Verification items for the finished model (mm, model axes). A direction names the side the tool comes from. Give positions to 0.01 mm unless a question says otherwise; leave off trailing zeros. Write each loop counter-clockwise with the first axis right and the second up, starting at its lowest first coordinate (ties: lowest second). Pieces come first, ordered by that corner, then holes.
Autodesk Inventor part; units mm, degrees
ref_plane "YZ Plane" through (0, 0, 0) normal (1, 0, 0) x (0, 1, 0)
ref_plane "XZ Plane" through (0, 0, 0) normal (0, 1, 0) x (-1, 0, 0)
ref_plane "XY Plane" through (0, 0, 0) normal (0, 0, 1) x (1, 0, 0)
sketch "Sketch1" plane through (0, 0, 0) normal (0, 0, 1) x (1, 0, 0)
  circle A0 centre (12.5, 11.5) radius 1.6
  line L0 (0, 0) -> (18, 0)
  line L1 (0, 0) -> (0, 3)
  arc A1 (18, 11.5) -> (7.7369, 14.25) centre (12.5, 11.5) ccw
  line L2 (12.5, 11.5) -> (7.7369, 14.25) construction
  line L3 (12.5, 11.5) -> (18, 11.5) construction
  line L4 (7.7369, 14.25) -> (0, 3)
  line L5 (18, 11.5) -> (18, 0)
  dimension "d17" = 3
  dimension "d19" = 11.5
  dimension "d23" = 90
  dimension "d25" = 12.5
  dimension "d31" = 5.5
  dimension "d32" = 150
  dimension "d49" = 3.2
extrude "Extrusion1" add sketch "Sketch1" along normal blind 4.5
sketch "Sketch4" plane through (0, 0, 4.5) normal (0, 0, 1) x (1, 0, 0)
  line L0 (0, 3) -> (0, 0)
  line L1 (18, 0) -> (18, 3)
  line L2 (0, 0) -> (18, 0)
  line L3 (18, 0) -> (18, 3)
  line L4 (18, 3) -> (0, 3)
  line L5 (0, 3) -> (0, 0)
  line L6 (18, 0) -> (18, 11.5)
extrude "Extrusion2" add sketch "Sketch4" along normal blind 4.5
sketch "Sketch5" plane through (0, 0, 0) normal (0, -1, 0) x (1, 0, 0)
  circle A0 centre (5, 5) radius 1.6
  circle A1 centre (15, 5) radius 1.6
  line L0 (0, 0) -> (18, 0)
  point P0 (20.0001, 0)
  dimension "d13" = 3.2
  dimension "d14" = 3.2
  dimension "d38" = 5
  dimension "d39" = 5
extrude "Extrusion3" cut sketch "Sketch5" against normal through all
sketch "Sketch6" plane through (0, 3, 9) normal (0, 1, 0) x (1, 0, 0)
  circle A0 centre (5, 4) radius 1.6
  circle A1 centre (5, 4) radius 3
  circle A2 centre (15, 4) radius 1.6
  circle A3 centre (15, 4) radius 3
  line L0 (0, 9) -> (18, 9)
  point P0 (20.0001, 9)
  dimension "d34" = 6
  dimension "d35" = 6
  dimension "d40" = 5
  dimension "d41" = 5
extrude "Extrusion4" cut sketch "Sketch6" along normal up to next
sketch "Sketch7" plane through (0, 0, 0) normal (0, -1, 0) x (1, 0, 0)
  line L0 (0, 0) -> (0, 9)
  line L1 (2.042, 0) -> (0, 0)
  line L2 (0, 0) -> (0, 9)
  line L3 (0, 9) -> (2.042, 9)
  line L4 (2.042, 9) -> (2.042, 0)
extrude "Extrusion5" cut sketch "Sketch7" against normal up to next
properties part number "lower_deck_shaft_mount_v3_for_AD"
Item 1: Scan lines: line 1 along Z through (x, y) = (15, 1.35); line 2 along Y through (x, z) = (12.5, 1.8); line 3 along Z through (x, y) = (11.25, 4.75). Record each from-to range of solid material in increasing order.
Answer key:
line 1: z = 0 to 3.4, 6.6 to 9
line 2: y = 0 to 9.9, 13.1 to 17
line 3: z = 0 to 4.5
Item 2: Depth check by flat-ended pin: pin 1 (3 mm diameter, centred on y = 10.5, z = 5.5, fed in from -X); pin 2 (4 mm diameter, centred on x = 4, z = 6, fed in from +Y); pin 3 (2 mm diameter, centred on x = 10, y = 13, fed in from +Z). Enter the tip coordinate at first touch or a pass-through.
Answer key:
pin 1: stops at x = 7.83
pin 2: stops at y = 3
pin 3: stops at z = 4.5
Item 3: Sectioned sample at C-C on y = 11. Record the cut outline in (x, z), then the cut area to 3 significant figures.
Answer key:
outline: (5.5, 0) - (10.98, 0) - (10.98, 4.5) - (7.96, 4.5) arc R3 cw to (5.5, 2.04) - close; (14.02, 0) - (18, 0) - (18, 4.5) - (17.96, 4.5) arc R3 cw to (14.02, 2.16) - close
area: 30.3 mm2
Item 4: Sectioned sample at D-D on y = 2.75. Record the cut outline in (x, z), then the cut area to 3 significant figures.
Answer key:
outline: (2.04, 0) - (18, 0) - (18, 9) - (2.04, 9) - close; hole circle Ø3.2 at (5, 5); hole circle Ø3.2 at (15, 5)
area: 128 mm2
Item 5: Sectioned sample at B-B on x = 12.5. Record the cut outline in (y, z).
Answer key:
outline: (0, 0) - (9.9, 0) - (9.9, 3.34) - (3, 3.34) - (3, 9) - (0, 9) - close; (13.1, 0) - (17, 0) - (17, 3.34) - (13.1, 3.34) - close
Item 6: Sectioned sample at A-A on z = 5.75. Record the cut outline in (x, y).
Answer key:
outline: (2.04, 0) - (3.59, 0) - (3.59, 3) - (2.04, 3) - close; (6.41, 0) - (13.59, 0) - (13.59, 3) - (6.41, 3) - close; (16.41, 0) - (18, 0) - (18, 3) - (16.41, 3) - close
Item 7: Set-up check for faces 1 (the face through (2.042, 2, 4)), 2 (the face through (10, 3, 6)), 3 (the face through (10, 10, 4.5)): record each of +Z, -Z, +X, -X, +Y, -Y from which the full face is reachable in a straight line by a thin tool's end or side.
Answer key:
face 1: +Z, -Z, -X, +Y, -Y
face 2: +Z, +Y
face 3: +Z, +X, -X, +Y
Item 8: Release check for a two-part mould opening along Z. For faces 4 (the face through (4.65, 1.48, 3.44)), 5 (the face through (13.4, 1.48, 5.07)), 6 (the face through (4.93, 10.17, 1.22)), 7 (the face through (5.864, 7.431, 2.127)) record: released by +Z, released by -Z, zero draft, split by the parting line, or undercut.
Answer key:
face 4: undercut
face 5: undercut
face 6: zero draft
face 7: released by +Z
